Here's the drawing with two shaded views (mm, measured from the low corner). I have some questions. Coordinates: 2 decimals unless noted, no trailing zeros. Loops run counter-clockwise (first coordinate to the right, second up) from the corner with the lowest first, then second, coordinate; pieces in that order, holes last. Notation, with made-up numbers: (85, -5) -> (144, -5) arc R6 cw to (144, 0) -> close; hole circle Ø8 at (18.25, 3). An arc over 180 degrees is marked (long way). Answer as a JSON object with one key per item and string values. Group by question number.
1) I want a section at B-B (x = 8). Write out the boundary of the cut face in (y, z).
2) If we mould it in two halves opening along Z, with no side actions, what happens to the marked faces 1, 2 and 3? For each: +Z half, -Z half, draft (parallel to the pull), parting line (faces both ways), or undercut.
3) I want a section at A-A (y = 8). Write out the boundary of the cut face in (x, z).
4) I'm going to push a flat-ended pin straight in: pin 1 (5 mm diameter, centred on x = 8, y = 62, fed in from +Z). Where does the tip first touch, or does it pass through?
5) I need wall thicknesses on probe 1 along X at (y, z) = (8, 45); probe 2 along Y at (x, z) = (57, 43); probe 3 along Z at (x, y) = (8.5, 6). Which ranges of each line are inside material? Lowest first, please. Write a range as [from, to].
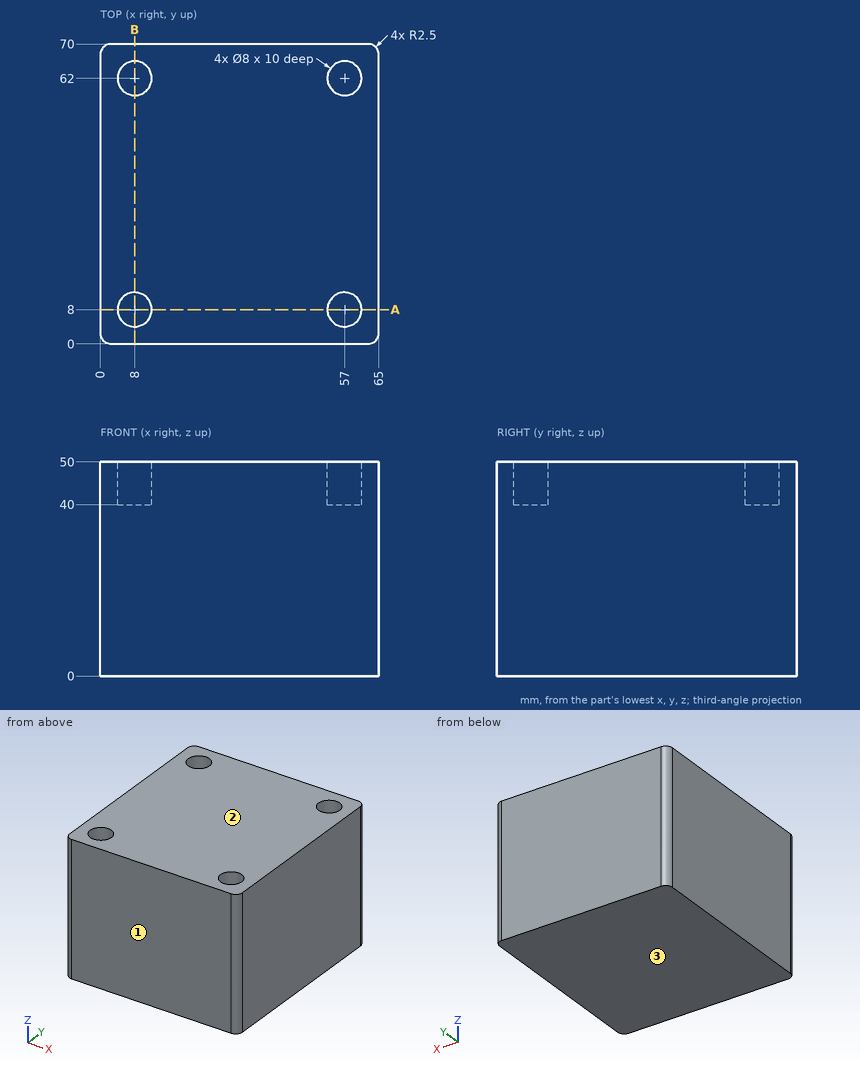
Determined:
{
 "1": {"outline": "(0, 0) -> (70, 0) -> (70, 50) -> (66, 50) -> (66, 40) -> (58, 40) -> (58, 50) -> (12, 50) -> (12, 40) -> (4, 40) -> (4, 50) -> (0, 50) -> close"},
 "2": {"face 1": "draft", "face 2": "+Z half", "face 3": "-Z half"},
 "3": {"outline": "(0, 0) -> (65, 0) -> (65, 50) -> (61, 50) -> (61, 40) -> (53, 40) -> (53, 50) -> (12, 50) -> (12, 40) -> (4, 40) -> (4, 50) -> (0, 50) -> close"},
 "4": {"pin 1": "z = 40"},
 "5": {"probe 1": "[0, 4], [12, 53], [61, 65]", "probe 2": "[0, 4], [12, 58], [66, 70]", "probe 3": "[0, 40]"}
}
